The listing builds one solid part. Answer for the finished solid, in the listing's coordinates (mm). Give positions to 0.01 mm unless a question says otherwise; leave off trailing zeros. Loops run counter-clockwise (first coordinate to the right, second up) from the corner with the lowest first, then second, coordinate; pieces in that order, holes last.
Item 1: Section C-C, the plane z = 0.5 is taken. Give the vertices of the cut face in (x, y).
Item 2: Consider line 1 along X through (y, z) = (-2.2, -9.5); line 2 along Z through (x, y) = (-8.5, -0.45); line 3 along X through (y, z) = (-1.95, -10.5). Determine where each line is inside the solid, lowest interval first.
Item 3: Section D-D, the plane x = 1.5 is taken. Give the vertices of the cut face in (y, z), and give its area (3 significant figures).
Item 4: Section A-A, the plane y = -1.35 is taken. Give the number of separate pieces and of enclosed holes in the cut face, and give its area (3 significant figures).
Item 5: The mould has two halves that part along Z. Classify faces 1 (the face through (-3, 0, -3)), 2 (the face through (-10.44, -1.48, -10.73)), 3 (the face through (-11.64, -1.52, -11.6)), 4 (the face through (-11.013, -1.479, 9.164)): pulls with the +Z half, pulls with the -Z half, needs draft (parallel to the pull), parting line crosses it, or undercut.
from build123d import *

# Parameters (mm, degrees)
SKETCH1_W           = 25
SKETCH1_H           = 25
SKETCH1_R           = 1.55
BOSS_EXTRUDE1_DEPTH = 3
FILLET1_R           = 25
FILLET2_R           = 3


with BuildPart() as part:
    # Sketch1 → Boss-Extrude1 (new body)
    with BuildSketch(Plane(origin=(0, 0, 0), x_dir=(1, 0, 0), z_dir=(0, 1, 0))):
        Rectangle(SKETCH1_W, SKETCH1_H)
        with Locations(Location((-9.5, 9.5, 0), (0, 0, 270))):
            Circle(SKETCH1_R, mode=Mode.SUBTRACT)
        with Locations(Location((-9.5, -9.5, 0), (0, 0, 270))):
            Circle(SKETCH1_R, mode=Mode.SUBTRACT)
    extrude(amount=-BOSS_EXTRUDE1_DEPTH)

    # Fillet1
    fillet1_edges = [part.edges().sort_by_distance(p)[0] for p in [
        (12.5, -1.5, 12.5),
    ]]
    fillet(fillet1_edges, radius=FILLET1_R - 0.0001)  # a hair under: the kernel refuses the full size

    # Fillet2
    fillet2_edges = [part.edges().sort_by_distance(p)[0] for p in [
        (-12.5, -1.5, 12.5),
        (-12.5, -1.5, -12.5),
        (12.5, -1.5, -12.5),
    ]]
    fillet(fillet2_edges, radius=FILLET2_R)


solid = part.part
Worked answers:
1. outline: (-12.5, -3) - (8.85, -3) - (8.85, 0) - (-12.5, 0) - close
2. line 1: x = -12.5 to -11.05, -7.95 to 12.29
2. line 2: z = -12.5 to -10.68, -8.32 to 8.32, 10.68 to 12.18
2. line 3: x = -12.33 to -10.68, -8.32 to 12.12
3. outline: (-3, -12.5) - (0, -12.5) - (0, 8.21) - (-3, 8.21) - close
3. area: 62.1 mm2
4. separate pieces: 1
4. enclosed holes: 2
4. area: 469 mm2
5. face 1: needs draft
5. face 2: undercut
5. face 3: pulls with the -Z half
5. face 4: undercut
